Input: part model. Units: mm. Frame: model coordinates. A direction names the side the tool comes from. Coordinates: 2 decimals unless noted, no trailing zeros. Loops run counter-clockwise (first coordinate to the right, second up) from the corner with the lowest first, then second, coordinate; pieces in that order, holes last.
```python
from build123d import *

# Parameters (mm, degrees)
SKETCH_1_W          = 117
SKETCH_1_H          = 45
SKETCH_1_R          = 7.25
EXTRUDE_1_DEPTH     = 13
SKETCH_2_W          = 108.5
SKETCH_2_H          = 35.5
CUT_EXTRUDE_1_DEPTH = 12
SKETCH_3_R          = 1.55
CUT_EXTRUDE_2_DEPTH = 6
SKETCH_4_W          = 50
SKETCH_4_H          = 10.556130204
CUT_EXTRUDE_3_DEPTH = 6
FILLET_1_R          = 2
FILLET_2_R          = 1


with BuildPart() as part:
    # 草图1 → 凸台-拉伸1 (new body)
    with BuildSketch(Plane.XY):
        Rectangle(SKETCH_1_W, SKETCH_1_H)
        with Locations(Location((-35, 0, 0), (0, 0, 180))):
            Circle(SKETCH_1_R, mode=Mode.SUBTRACT)
        with Locations(Location((35, 0, 0), (0, 0, 180))):
            Circle(SKETCH_1_R, mode=Mode.SUBTRACT)
    extrude(amount=EXTRUDE_1_DEPTH)

    # 草图2 → 切除-拉伸1 (cut)
    with BuildSketch(Plane.XY.offset(13)):
        Rectangle(SKETCH_2_W, SKETCH_2_H)
    extrude(amount=-CUT_EXTRUDE_1_DEPTH, mode=Mode.SUBTRACT)

    # 草图3 → 切除-拉伸2 (cut)
    with BuildSketch(Plane.XY.offset(13)):
        with Locations((-56, 20)):
            Circle(SKETCH_3_R)
        with Locations(Location((-56, -20, 0), (0, 0, 180))):
            Circle(SKETCH_3_R)
        with Locations((56, -20)):
            Circle(SKETCH_3_R)
        with Locations(Location((56, 20, 0), (0, 0, 180))):
            Circle(SKETCH_3_R)
    extrude(amount=-CUT_EXTRUDE_2_DEPTH, mode=Mode.SUBTRACT)

    # 草图4 → 切除-拉伸3 (cut)
    with BuildSketch(Plane.XY.offset(13)):
        with Locations((0, -20)):
            Rectangle(SKETCH_4_W, SKETCH_4_H)
    extrude(amount=-CUT_EXTRUDE_3_DEPTH, mode=Mode.SUBTRACT)

    # 圆角1
    fillet_1_edges = [part.edges().sort_by_distance(p)[0] for p in [
        (58.5, -22.5, 6.5),
        (-58.5, -22.5, 6.5),
        (-58.5, 22.5, 6.5),
        (58.5, 22.5, 6.5),
    ]]
    fillet(fillet_1_edges, radius=FILLET_1_R)

    # 圆角2
    fillet_2_edges = [part.edges().sort_by_distance(p)[0] for p in [
        (0, -17.75, 7),
        (25, -17.75, 10),
        (-25, -17.75, 10),
        (-25, -22.5, 10),
        (25, -22.5, 10),
        (0, -22.5, 7),
        (-25, -20.125, 13),
        (25, -20.125, 13),
    ]]
    fillet(fillet_2_edges, radius=FILLET_2_R)


solid = part.part
```
Item 1: Reachability of faces 4 (the face through (-57.93, -21.9, 6.59)), 5 (the face through (25, -20, 10)), 6 (the face through (-56, 20, 7)) from +Z, -Z, +X, -X, +Y, -Y: full face, straight path, thin tool, end or side. Return the list, or none.
Result:
face 4: +Z, -Z, -X, -Y
face 5: +Z, -Y
face 6: +Z
Item 2: Contact query for flat-ended pins moving along their axis: P1, Ø1.5, axis at x = 55.5, y = -20, coming from the +Z side; P2, Ø8, axis at x = 36, y = -6.5, coming from the +Z side. Output: stop coordinate, or through.
Result:
P1: stops at z = 7
P2: stops at z = 1
Item 3: Line query: L1, parallel to Y at x = -56, z = 9.5; L2, parallel to Y at x = 47.5, z = 2.5; L3, parallel to X at y = -2, z = 5. Output: solid intervals per line, ascending.
Result:
L1: y = -22.5 to -21.55, -18.45 to 18.45, 21.55 to 22.5
L2: y = -22.5 to -17.75, 17.75 to 22.5
L3: x = -58.5 to -54.25, 54.25 to 58.5
Item 4: Section query A-A (z = 8.5). Output: boundary loops of the cut face in (x, y).
Result:
outline: (-58.5, -20.5) arc R2 ccw to (-56.5, -22.5) - (-26, -22.5) arc R1 ccw to (-25, -21.5) - (-25, -18.75) arc R1 ccw to (-26, -17.75) - (-54.25, -17.75) - (-54.25, 17.75) - (54.25, 17.75) - (54.25, -17.75) - (26, -17.75) arc R1 ccw to (25, -18.75) - (25, -21.5) arc R1 ccw to (26, -22.5) - (56.5, -22.5) arc R2 ccw to (58.5, -20.5) - (58.5, 20.5) arc R2 ccw to (56.5, 22.5) - (-56.5, 22.5) arc R2 ccw to (-58.5, 20.5) - close; hole circle Ø3.1 at (-56, -20); hole circle Ø3.1 at (-56, 20); hole circle Ø3.1 at (56, -20); hole circle Ø3.1 at (56, 20)
Item 5: Section query C-C (z = 3.25). Output: boundary loops of the cut face in (x, y).
Result:
outline: (-58.5, -20.5) arc R2 ccw to (-56.5, -22.5) - (56.5, -22.5) arc R2 ccw to (58.5, -20.5) - (58.5, 20.5) arc R2 ccw to (56.5, 22.5) - (-56.5, 22.5) arc R2 ccw to (-58.5, 20.5) - close; hole (-54.25, -17.75) - (54.25, -17.75) - (54.25, 17.75) - (-54.25, 17.75) - close
Item 6: Section query B-B (x = 35). Output: boundary loops of the cut face in (y, z), then the cut area to 4 significant figures.
Result:
outline: (-22.5, 0) - (-7.25, 0) - (-7.25, 1) - (-17.75, 1) - (-17.75, 13) - (-22.5, 13) - close; (7.25, 0) - (22.5, 0) - (22.5, 13) - (17.75, 13) - (17.75, 1) - (7.25, 1) - close
area: 144.5 mm2
Item 7: Section query D-D (x = 50.5). Output: boundary loops of the cut face in (y, z), then the cut area to 3 significant figures.
Result:
outline: (-22.5, 0) - (22.5, 0) - (22.5, 13) - (17.75, 13) - (17.75, 1) - (-17.75, 1) - (-17.75, 13) - (-22.5, 13) - close
area: 159 mm2
Item 8: Mould query, pull axis X, two halves, no side actions, for faces 1 (the face through (56, 20, 7)), 2 (the face through (-58.5, 0, 6)), 3 (the face through (57.9, 21.93, 6.59)). Classes: +X half, -X half, draft (parallel to the pull), parting line (faces both ways), or undercut.
Result:
face 1: undercut
face 2: -X half
face 3: +X half
